Model file for the job. Use its own axes, mm. A direction names the side the tool comes from. Coordinates: 2 decimals unless noted, no trailing zeros. Write each loop counter-clockwise with the first axis right and the second up, starting at its lowest first coordinate (ties: lowest second). Pieces come first, ordered by that corner, then holes. Notation, with made-up numbers: M -36,84.5 L -5,84.5 A12 ccw -5,107.5 Z; hole C 53.25,63 d3. An arc over 180 degrees is marked long. One line per question, with ' | ' between items. Start each with the question number.
(1) Cut at B-B (x = 11). Write the cut outline in (y, z), plus the area to 3 significant figures.
(2) Tool access for faces 1 (the face through (1, -101, 13)), 2 (the face through (20, -58, 24.8)): list every direction of +Z, -Z, +X, -X, +Y, -Y with a clear straight run to the whole face (end or side of a thin tool).
(3) Cut at A-A (z = 7). Write the cut outline in (x, y).
(4) Cut at C-C (y = -95). Write the cut outline in (x, z), plus the area to 3 significant figures.
(5) Wall check: probe 1 along Y at (x, z) = (13.5, 22.5); probe 2 along X at (y, z) = (-50, 15); probe 3 along Z at (x, y) = (21, -69). Give the ranges that are in metal, low to high.
(6) Two-plate mould, pull along Y, no slides. Class faces 3 (the face through (22, -57, 0)), 4 (the face through (22, -101, 1)): +Y half, -Y half, draft (parallel to the pull), parting line (faces both ways), or undercut.
(7) Flat gauge pins, fed straight in: pin 1 Ø8 at (x, y) = (16, -25) entering from -Z; pin 2 Ø9 at (x, y) = (12.5, -6) entering from +Z. Where does each tip first touch, or does it go through?
from build123d import *

# Parameters (mm, degrees)
F0_W     = 43.8
F0_H     = 115.8
F1_DEPTH = 1
F2_W     = 41.8
F2_H     = 1
F3_DEPTH = 23.8


# Not quite as in the source:
# - a feature names something its author has since deleted; it is built from what else it names


with BuildPart() as f1:
    # F0 (on Top) → F1 (new body)
    with BuildSketch(Plane.XY):
        with Locations((21.9, -57.9)):
            Rectangle(F0_W, F0_H)
    extrude(amount=F1_DEPTH)

    # F2 (on face) → F3 (join)
    with BuildSketch(Plane.XY.offset(1)):
        Polygon((0, -114.8), (0, -115.8), (43.8, -115.8), (43.8, -114.8), (42.8, -114.8), (1, -114.8), align=None)
        Polygon((0, 0), (0, -114.8), (1, -114.8), (1, -87.35), (1, -87.1), (1, -86.35), (1, -86.1), (1, -58.4), (1, -57.4), (1, -39.1), (1, -38.1), (1, -19.8), (1, -18.8), (1, -1), (1, 0), align=None)
        Polygon((42.8, -114.8), (43.8, -114.8), (43.8, 0), (42.8, 0), (42.8, -1), (42.8, -18.8), (42.8, -19.8), (42.8, -38.1), (42.8, -39.1), (42.8, -57.4), (42.8, -58.4), (42.8, -86.1), (42.8, -87.1), align=None)
        with Locations((21.9, -0.5)):
            Rectangle(F2_W, F2_H)
        with Locations((21.9, -19.3)):
            Rectangle(F2_W, F2_H)
        with Locations((21.9, -38.6)):
            Rectangle(F2_W, F2_H)
        with Locations((21.9, -57.9)):
            Rectangle(F2_W, F2_H)
        Polygon((1, -87.1), (42.8, -87.1), (42.8, -86.1), (1, -86.1), (1, -86.35), align=None)
    extrude(amount=F3_DEPTH)


solid = f1.part
Filled in:
1) outline: M -115.8,0 L 0,0 L 0,24.8 L -1,24.8 L -1,1 L -18.8,1 L -18.8,24.8 L -19.8,24.8 L -19.8,1 L -38.1,1 L -38.1,24.8 L -39.1,24.8 L -39.1,1 L -57.4,1 L -57.4,24.8 L -58.4,24.8 L -58.4,1 L -86.1,1 L -86.1,24.8 L -87.1,24.8 L -87.1,1 L -114.8,1 L -114.8,24.8 L -115.8,24.8 Z | area: 259 mm²
2) face 1: +Z | face 2: +Z, +X, -X, +Y, -Y
3) outline: M 0,-115.8 L 43.8,-115.8 L 43.8,0 L 0,0 Z; hole M 1,-114.8 L 42.8,-114.8 L 42.8,-87.1 L 1,-87.1 Z; hole M 1,-86.1 L 42.8,-86.1 L 42.8,-58.4 L 1,-58.4 Z; hole M 1,-57.4 L 42.8,-57.4 L 42.8,-39.1 L 1,-39.1 Z; hole M 1,-38.1 L 42.8,-38.1 L 42.8,-19.8 L 1,-19.8 Z; hole M 1,-18.8 L 42.8,-18.8 L 42.8,-1 L 1,-1 Z
4) outline: M 0,0 L 43.8,0 L 43.8,24.8 L 42.8,24.8 L 42.8,1 L 1,1 L 1,24.8 L 0,24.8 Z | area: 91.4 mm²
5) probe 1: -115.8 to -114.8, -87.1 to -86.1, -58.4 to -57.4, -39.1 to -38.1, -19.8 to -18.8, -1 to 0 | probe 2: 0 to 1, 42.8 to 43.8 | probe 3: 0 to 1
6) face 3: draft | face 4: undercut
7) pin 1: z = 0 | pin 2: z = 1
